```python
from build123d import *

# Parameters (mm, degrees)
SKETCH_W             = 162
SKETCH_H             = 33.9
PAD_DEPTH            = 3
POCKET_DEPTH         = 81.001
POCKET_DEPTH_BACK    = 81.001
POCKET001_DEPTH      = 81.001
POCKET001_DEPTH_BACK = 81.001


with BuildPart() as part:
    # Sketch → Pad (new body)
    with BuildSketch(Plane.XY):
        Rectangle(SKETCH_W, SKETCH_H)
    extrude(amount=PAD_DEPTH)

    # Sketch001 → Pocket (cut, two sides)
    with BuildSketch(Plane.YZ) as pocket_sk:
        Polygon((15.47, 3), (16.95, 3), (16.95, 0), (15.47, 1), align=None)
    extrude(amount=-POCKET_DEPTH, mode=Mode.SUBTRACT)
    extrude(pocket_sk.sketch, amount=POCKET_DEPTH_BACK, mode=Mode.SUBTRACT)

    # MirroredSketch → Pocket001 (cut, two sides)
    with BuildSketch(Plane.YZ) as pocket001_sk:
        Polygon((-15.47, 3), (-16.95, 3), (-16.95, 0), (-15.47, 1), align=None)
    extrude(amount=-POCKET001_DEPTH, mode=Mode.SUBTRACT)
    extrude(pocket001_sk.sketch, amount=POCKET001_DEPTH_BACK, mode=Mode.SUBTRACT)


solid = part.part
```
Source: CAD feature listing. Evaluate the final solid. Frame: model axes, mm. Give positions to 0.01 mm unless a question says otherwise; leave off trailing zeros. Write each loop counter-clockwise with the first axis right and the second up, starting at its lowest first coordinate (ties: lowest second). Pieces come first, ordered by that corner, then holes.
1. Section query B-B (z = 1.95). Return the cut outline in (x, y).
2. First-contact query: pin 1 (1 mm diameter, centred on x = 8, z = 2.5, fed in from +Y); pin 2 (1.6 mm diameter, centred on x = -6, z = 1.5, fed in from -Y). Flat tips, straight axial feed; report the tip coordinate or a pass-through.
3. Section query A-A (x = -62.5). Return the cut outline in (y, z), then the cut area to 3 significant figures.
4. Material intervals for line 1 along Y through (x, z) = (-27.5, 2.8); line 2 along Y through (x, z) = (70.5, 0.75), sorted ascending.
Output values:
1. outline: (-81, -15.47) - (81, -15.47) - (81, 15.47) - (-81, 15.47) - close
2. pin 1: stops at y = 15.47
2. pin 2: stops at y = -15.91
3. outline: (-16.95, 0) - (16.95, 0) - (15.47, 1) - (15.47, 3) - (-15.47, 3) - (-15.47, 1) - close
3. area: 94.3 mm2
4. line 1: y = -15.47 to 15.47
4. line 2: y = -15.84 to 15.84
